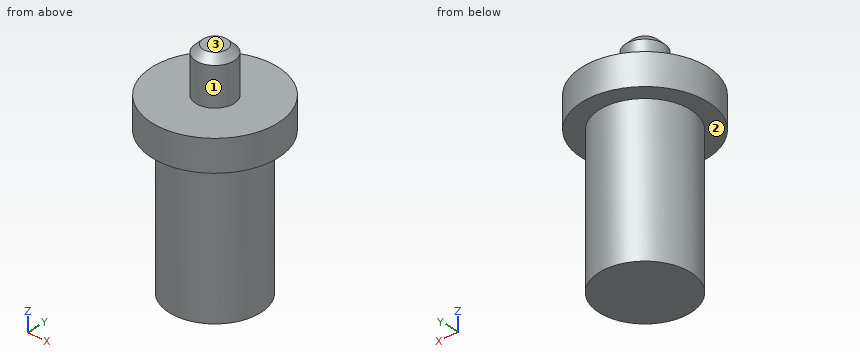
```python
from build123d import *

# Parameters (mm, degrees)
SKETCH1_R           = 3.45
BOSS_EXTRUDE1_DEPTH = 1.72
SKETCH2_R           = 2.5
BOSS_EXTRUDE2_DEPTH = 8
SKETCH3_R           = 1.05
BOSS_EXTRUDE3_DEPTH = 2.5
CHAMFER1_SIZE       = 0.4


with BuildPart() as part:
    # Sketch1 → Boss-Extrude1 (new body)
    with BuildSketch(Plane.XY):
        Circle(SKETCH1_R)
    extrude(amount=-BOSS_EXTRUDE1_DEPTH)

    # Sketch2 → Boss-Extrude2 (add)
    with BuildSketch(Plane(origin=(0, 0, -1.72), x_dir=(-1, 0, 0), z_dir=(0, 0, -1))):
        with Locations(Location((0, 0, 0), (0, 0, 180))):
            Circle(SKETCH2_R)
    extrude(amount=BOSS_EXTRUDE2_DEPTH)

    # Sketch3 → Boss-Extrude3 (add)
    with BuildSketch(Plane.XY):
        Circle(SKETCH3_R)
    extrude(amount=BOSS_EXTRUDE3_DEPTH)

    # Chamfer1
    chamfer1_edges = [part.edges().sort_by_distance(p)[0] for p in [
        (-1.05, 0, 2.5),
    ]]
    chamfer(chamfer1_edges, length=CHAMFER1_SIZE)


solid = part.part
```
CAD build for the part. Positions are in the model's coordinates, mm. Face numbers are marked on the shaded views. A direction names the side the tool comes from. Give positions to 0.01 mm unless a question says otherwise; leave off trailing zeros. Loops run counter-clockwise (first coordinate to the right, second up) from the corner with the lowest first, then second, coordinate; pieces in that order, holes last. Notation, with made-up numbers: (-16.75, 35.5) -> (29.25, 35.5) arc R14 ccw to (29.25, 45.5) -> close; hole circle Ø3 at (-30.75, -39). An arc over 180 degrees is marked (long way). Use a Markdown table: item, result.
1. Wall check: L1, parallel to Z at x = 1.25, y = 2.5; L2, parallel to Z at x = -2.25, y = -0.5; L3, parallel to X at y = 0.75, z = -5.5. Give the ranges that are in metal, low to high. Write a range as [from, to].
Check result:
| item | result |
|---|---|
| L1 | z = [-1.72, 0] |
| L2 | z = [-9.72, 0] |
| L3 | x = [-2.38, 2.38] |
2. Slice it at C-C (z = -0.5). List the corners of the cut face in (x, y).
Check result:
| item | result |
|---|---|
| outline | circle Ø6.9 at (0, 0) |
3. Slice it at D-D (y = 1.75). List the corners of the cut face in (x, z), plus the area to 3 significant figures.
Check result:
| item | result |
|---|---|
| outline | (-2.97, -1.72) -> (-1.79, -1.72) -> (-1.79, -9.72) -> (1.79, -9.72) -> (1.79, -1.72) -> (2.97, -1.72) -> (2.97, 0) -> (-2.97, 0) -> close |
| area | 38.8 mm^2 |
4. Flat gauge pins, fed straight in: pin 1 (1.5 mm diameter, centred on x = 1.5, z = -1, fed in from -Y); pin 2 (1.5 mm diameter, centred on y = -1, z = -1.5, fed in from -X); pin 3 (3 mm diameter, centred on y = -0.5, z = -8.5, fed in from -X). Where does each tip first touch, or does it go through?
Check result:
| item | result |
|---|---|
| pin 1 | stops at y = -3.37 |
| pin 2 | stops at x = -3.44 |
| pin 3 | stops at x = -2.5 |
5. Which spindle directions (+Z, -Z, +X, -X, +Y, -Y) get a long thin tool onto all of the face, cutting with end or side? Do the marked faces 1, 2 and 3. Say none if no direction does.
Check result:
| item | result |
|---|---|
| face 1 | +Z |
| face 2 | -Z |
| face 3 | +Z, +X, -X, +Y, -Y |
6. Slice it at A-A (y = 0). List the corners of the cut face in (x, z).
Check result:
| item | result |
|---|---|
| outline | (-3.45, -1.72) -> (-2.5, -1.72) -> (-2.5, -9.72) -> (2.5, -9.72) -> (2.5, -1.72) -> (3.45, -1.72) -> (3.45, 0) -> (1.05, 0) -> (1.05, 2.1) -> (0.65, 2.5) -> (-0.65, 2.5) -> (-1.05, 2.1) -> (-1.05, 0) -> (-3.45, 0) -> close |
